Model file for the job. Use its own axes, mm. A direction names the side the tool comes from. Coordinates: 2 decimals unless noted, no trailing zeros. Order: outer loops, then holes, each group sorted by start corner. A loop starts at its lowest first (then second) coordinate and runs counter-clockwise, first axis right, second up. Notation, with made-up numbers: (62, 31) -> (89, 31) arc R34 ccw to (89, 66) -> close; hole circle Ø9 at (85, 6). An arc over 180 degrees is marked (long way). Return JSON: item names as keys, results as strings. Group by question number.
1) Cut at B-B (z = 50). Write the cut outline in (x, y), and give its area (3 significant figures).
2) Cut at A-A (z = 25). State how many separate pieces and enclosed holes the cut face has, and give its area (3 significant figures).
3) Pull direction Y, two halves, no side cores. Call faces 1 (the flat face through (77, 168, 41.5)), 2 (the flat face through (46, 168, 20)), 3 (the cylindrical face through (206.93, 72.13, 33.96)): +Y half, -Y half, draft (parallel to the pull), parting line (faces both ways), or undercut.
4) Probe line 1 (X direction, y = 200, z = 32); line 2 (Y direction, x = 125, z = 27); line 3 (X direction, y = 186, z = 38). List the from-to ranges inside material, lowest first.
5) Flat gauge pins, fed straight in: pin 1 (11 mm diameter, centred on x = 60, z = 28.5, fed in from +Y); pin 2 (3 mm diameter, centred on x = 62.5, y = 129.5, fed in from -Z); pin 3 (4 mm diameter, centred on x = 109, y = 186.5, fed in from +Z); pin 4 (2 mm diameter, centred on x = 128, z = 26.5, fed in from -Y). Where does each tip first touch, or does it go through?
6) Which spindle directions (+Z, -Z, +X, -X, +Y, -Y) get a long thin tool onto all of the face, cutting with end or side? Do faces 4 (the flat face through (69, 190, 36)), 5 (the cylindrical face through (129.032, 206.324, 33.964)), 6 (the flat face through (81, 168, 35.5)), 7 (the flat face through (40, 168, 23)). Say none if no direction does.
from build123d import *

# Parameters (mm, degrees)
SKETCH027_R      = 1.625
SKETCH027_R_2    = 2
SKETCH027_R_3    = 2.8
SKETCH027_R_4    = 1.65
EXTRUDE004_DEPTH = 80
EXTRUDE003_DEPTH = 45
SKETCH025_W      = 275
SKETCH025_H      = 275
EXTRUDE002_DEPTH = 5
SKETCH023_W      = 275
SKETCH023_H      = 275
SKETCH024_W      = 0.1
SKETCH024_H      = 0.1
SKETCH_R         = 7.5
EXTRUDE001_DEPTH = 63.75


with BuildPart() as extrude004:
    # Sketch027 → Extrude004 (new body)
    with BuildSketch(Plane.XY):
        with Locations((51.75, 92.5)):
            Circle(SKETCH027_R)
        with Locations((87.75, 108.5)):
            Circle(SKETCH027_R)
        with Locations((121.75, 185.5)):
            Circle(SKETCH027_R_2)
        with Locations((147.3, 147.75)):
            Circle(SKETCH027_R)
        with Locations((218.8, 147.75)):
            Circle(SKETCH027_R)
        with Locations((218.8, 219.25)):
            Circle(SKETCH027_R)
        with Locations((147.3, 219.25)):
            Circle(SKETCH027_R)
        with Locations((75, 200)):
            Circle(SKETCH027_R_3)
        with Locations((125, 200)):
            Circle(SKETCH027_R_3)
        with Locations((200, 75)):
            Circle(SKETCH027_R_3)
        with Locations((75, 75)):
            Circle(SKETCH027_R_3)
        with Locations((91, 186.5)):
            Circle(SKETCH027_R_4)
        with Locations((109, 186.5)):
            Circle(SKETCH027_R_4)
        with Locations((91, 151.5)):
            Circle(SKETCH027_R_4)
        with Locations((109, 151.5)):
            Circle(SKETCH027_R_4)
    extrude(amount=EXTRUDE004_DEPTH)


with BuildPart() as extrude003:
    # Sketch026 → Extrude003 (new body)
    with BuildSketch(Plane.XZ):
        Polygon((46, 5), (40, 5), (40, 41.5), (115, 41.5), (115, 35.5), (46, 35.5), align=None)
    extrude(amount=EXTRUDE003_DEPTH)


with BuildPart() as extrude003_1:
    # Extrude003 placement: moved
    add(extrude003.part.moved(Location((0, 190, 0))))


with BuildPart() as level01s001:
    # Sketch025 → Extrude002 (new body)
    with BuildSketch(Plane.XY):
        with Locations((137.5, 137.5)):
            Rectangle(SKETCH025_W, SKETCH025_H)
    extrude(amount=EXTRUDE002_DEPTH)


with BuildPart() as baselevel:
    # Sketch023 → Loft004 section 0
    with BuildSketch(Plane.XY):
        with Locations((137.5, 137.5)):
            Rectangle(SKETCH023_W, SKETCH023_H)
    # Sketch024 → Loft004 section 1
    with BuildSketch(Plane.XY.offset(175.1)):
        with Locations((137.5, 137.5)):
            Rectangle(SKETCH024_W, SKETCH024_H)
    loft()


with BuildPart() as baselevel_1:
    # Loft004 placement: moved
    add(baselevel.part.moved(Location((0, 0, -8.25))))

    # Common001: intersect level01s001
    add(level01s001.part, mode=Mode.INTERSECT)


with BuildPart() as level02:
    # Sketch → Extrude001 (new body)
    with BuildSketch(Plane.XY):
        with Locations((75, 200)):
            Circle(SKETCH_R)
        with Locations((125, 200)):
            Circle(SKETCH_R)
        with Locations((75, 75)):
            Circle(SKETCH_R)
        with Locations((200, 75)):
            Circle(SKETCH_R)
    extrude(amount=EXTRUDE001_DEPTH)

    # Fusion: union BaseLevel
    add(baselevel_1.part)

    # Fusion056: union Extrude003
    add(extrude003_1.part)

    # Cut001: cut Extrude004
    add(extrude004.part, mode=Mode.SUBTRACT)


solid = level02.part
Answers below:
{
 "1": {"outline": "circle Ø15 at (75, 75); circle Ø15 at (75, 200); circle Ø15 at (125, 200); circle Ø15 at (200, 75); hole circle Ø5.6 at (75, 75); hole circle Ø5.6 at (75, 200); hole circle Ø5.6 at (125, 200); hole circle Ø5.6 at (200, 75)", "area": "608 mm^2"},
 "2": {"separate pieces": "5", "enclosed holes": "4", "area": "878 mm^2"},
 "3": {"face 1": "undercut", "face 2": "draft", "face 3": "parting line"},
 "4": {"line 1": "x = 67.5 to 72.2, 77.8 to 82.5, 117.5 to 122.2, 127.8 to 132.5", "line 2": "y = 192.5 to 197.2, 202.8 to 207.5", "line 3": "x = 40 to 89.43, 92.57 to 107.43, 110.57 to 115"},
 "5": {"pin 1": "passes through", "pin 2": "stops at z = 0", "pin 3": "stops at z = 41.5", "pin 4": "stops at y = 192.77"},
 "6": {"face 4": "+Z, +X, -X", "face 5": "+Z", "face 6": "+X", "face 7": "+Z, -X, +Y, -Y"}
}
